Autodesk Inventor part; units mm, degrees
ref_plane "YZ Plane" through (0, 0, 0) normal (1, 0, 0) x (0, 1, 0)
ref_plane "XZ Plane" through (0, 0, 0) normal (0, 1, 0) x (-1, 0, 0)
ref_plane "XY Plane" through (0, 0, 0) normal (0, 0, 1) x (1, 0, 0)
sketch "草圖1" plane through (0, 0, 0) normal (0, 0, 1) x (1, 0, 0)
  line L0 (0, 0) -> (0, 7)
  line L1 (0, 7) -> (3.3317, 9.2136)
  line L2 (3.3317, 9.2136) -> (4.2133, 8)
  line L3 (4.2133, 8) -> (4.2133, 0)
  line L4 (4.2133, 0) -> (0, 0)
  dimension "d0" = 7
  dimension "d1" = 4
  dimension "d2" = 1.5
  dimension "d3" = 8
extrude "擠出1" add sketch "草圖1" along normal blind 5.3
sketch "草圖2" plane through (0, 0, 0) normal (-1, 0, 0) x (0, 0, 1)
  line L0 (1, 2.25) -> (4.3, 2.25)
  line L1 (4.4, 2.35) -> (4.4, 5.65)
  line L2 (4.3, 5.75) -> (1, 5.75)
  line L3 (0.9, 5.65) -> (0.9, 2.35)
  line L4 (0.9, 2.25) -> (4.4, 5.75) construction
  line L5 (4.4, 2.25) -> (0.9, 5.75) construction
  line L6 (1.2, 5.55) -> (2.2, 5.55)
  line L7 (2.3, 5.45) -> (2.3, 4.45)
  line L8 (2.2, 4.35) -> (1.2, 4.35)
  line L9 (1.1, 4.45) -> (1.1, 5.45)
  line L10 (1.1, 5.55) -> (2.3, 4.35) construction
  line L11 (2.3, 5.55) -> (1.1, 4.35) construction
  line L12 (3.1, 4.35) -> (4.1, 4.35)
  line L13 (4.2, 4.45) -> (4.2, 5.45)
  line L14 (4.1, 5.55) -> (3.1, 5.55)
  line L15 (3, 5.45) -> (3, 4.45)
  line L16 (3, 4.35) -> (4.2, 5.55) construction
  line L17 (4.2, 4.35) -> (3, 5.55) construction
  line L18 (3.1, 3.65) -> (4.1, 3.65)
  line L19 (4.2, 3.55) -> (4.2, 2.55)
  line L20 (4.1, 2.45) -> (3.1, 2.45)
  line L21 (3, 2.55) -> (3, 3.55)
  line L22 (3, 3.65) -> (4.2, 2.45) construction
  line L23 (4.2, 3.65) -> (3, 2.45) construction
  line L24 (1.2, 2.45) -> (2.2, 2.45)
  line L25 (2.3, 2.55) -> (2.3, 3.55)
  line L26 (2.2, 3.65) -> (1.2, 3.65)
  line L27 (1.1, 3.55) -> (1.1, 2.55)
  line L28 (1.1, 2.45) -> (2.3, 3.65) construction
  line L29 (2.3, 2.45) -> (1.1, 3.65) construction
  arc A0 (1, 5.75) -> (0.9, 5.65) centre (1, 5.65) ccw
  arc A1 (0.9, 2.35) -> (1, 2.25) centre (1, 2.35) ccw
  arc A2 (4.3, 2.25) -> (4.4, 2.35) centre (4.3, 2.35) ccw
  arc A3 (4.4, 5.65) -> (4.3, 5.75) centre (4.3, 5.65) ccw
  arc A4 (4.2, 5.45) -> (4.1, 5.55) centre (4.1, 5.45) ccw
  arc A5 (4.1, 4.35) -> (4.2, 4.45) centre (4.1, 4.45) ccw
  arc A6 (3, 4.45) -> (3.1, 4.35) centre (3.1, 4.45) ccw
  arc A7 (3.1, 5.55) -> (3, 5.45) centre (3.1, 5.45) ccw
  arc A8 (2.3, 5.45) -> (2.2, 5.55) centre (2.2, 5.45) ccw
  arc A9 (1.2, 5.55) -> (1.1, 5.45) centre (1.2, 5.45) ccw
  arc A10 (1.1, 4.45) -> (1.2, 4.35) centre (1.2, 4.45) ccw
  arc A11 (2.2, 4.35) -> (2.3, 4.45) centre (2.2, 4.45) ccw
  arc A12 (2.3, 3.55) -> (2.2, 3.65) centre (2.2, 3.55) ccw
  arc A13 (2.2, 2.45) -> (2.3, 2.55) centre (2.2, 2.55) ccw
  arc A14 (1.1, 2.55) -> (1.2, 2.45) centre (1.2, 2.55) ccw
  arc A15 (1.2, 3.65) -> (1.1, 3.55) centre (1.2, 3.55) ccw
  arc A16 (3.1, 3.65) -> (3, 3.55) centre (3.1, 3.55) ccw
  arc A17 (4.2, 3.55) -> (4.1, 3.65) centre (4.1, 3.55) ccw
  arc A18 (4.1, 2.45) -> (4.2, 2.55) centre (4.1, 2.55) ccw
  arc A19 (3, 2.55) -> (3.1, 2.45) centre (3.1, 2.55) ccw
  point P0 (2.65, 4)
  point P1 (1.7, 4.95)
  point P2 (3.6, 4.95)
  point P3 (3.6, 3.05)
  point P4 (1.7, 3.05)
  dimension "d7" = 3.5
  dimension "d8" = 3.5
  dimension "d9" = 1.2
  dimension "d10" = 1.2
  dimension "d11" = 0.2
  dimension "d12" = 0.1
  dimension "d13" = 0.1
extrude "擠出2" add sketch "草圖2" along normal blind 0.2
extrude "擠出3" cut sketch "草圖2" against normal blind 0.1 contours L6 A8 L7 A11 L8 A10 L9 A9 | A6 L15 A7 L14 A4 L13 A5 L12 | L18 A17 L19 A18 L20 A19 L21 A16 | A14 L27 A15 L26 A12 L25 A13 L24
sketch "草圖3" plane through (0, 0, 0) normal (0, -1, 0) x (1, 0, 0)
  line L0 (4.2133, 0) -> (4.2133, 5.3)
  line L1 (4.2133, 0.2) -> (0.2, 0.2)
  line L2 (0.2, 0.2) -> (0.2, 5.1)
  line L3 (0.2, 5.1) -> (4.2133, 5.1)
  line L4 (4.2133, 5.1) -> (4.2133, 0.2)
  line L5 (0, 0) -> (4.2133, 0)
  line L6 (0, 0) -> (0, 5.3)
  line L7 (0, 5.3) -> (4.2133, 5.3)
  dimension "d18" = 0.2
  dimension "d19" = 0.2
  dimension "d20" = 0.2
extrude "擠出4" add sketch "草圖3" along normal blind 3 contours L1 L2 L3 L0
sketch "草圖4" plane through (0.2, 0, 5.1) normal (0, 0, 1) x (1, 0, 0)
  line L0 (4.0133, 0) -> (0, 0)
  line L1 (0, 0) -> (4.0133, -3)
  line L2 (0, -3) -> (4.0133, -3)
  line L3 (4.0133, -3) -> (0, -3)
  line L4 (0, -3) -> (0, 0)
  point P0 (-0.2, 0)
extrude "擠出5" cut sketch "草圖4" against normal up to surface (4.9 mm away)
properties part number "頭 小小屋"
Design review of the part built by this model. Coordinates are the model's own, in mm. A direction names the side the tool comes from. Round coordinates to 2 decimals unless told otherwise and drop trailing zeros. Write each loop counter-clockwise with the first axis right and the second up, starting at its lowest first coordinate (ties: lowest second). Pieces come first, ordered by that corner, then holes. Notation, with made-up numbers: (17, -1.75) - (32, -1.75) arc R22 ccw to (32, 17.25) - close; hole circle Ø8 at (83, 8.5). An arc over 180 degrees is marked (long way). Use a Markdown table: item, result. Add a question column.
1. Wall thickness on probe 1 along Y at (x, z) = (0.05, 1.8); probe 2 along X at (y, z) = (5.25, 4.6); probe 3 along Z at (x, y) = (2.7, -0.25): over which ranges is each line inside the solid? List them lowest first.
2. We need section B-B (z = 3.8). State the section outline as (x, y) points, then the cut area to 3 significant figures.
3. For faces 4 (the face through (0.1, 3, 4)), 5 (the face through (3, -1, 0.2)), 6 (the face through (3, -1, 5.1)), list the 3-axis set-ups (+Z, -Z, +X, -X, +Y, -Y) from which the entire face can be reached by the end or side of a thin tool; tool diameter is ignored.
4. We need section A-A (y = 5.25). State the section outline as (x, z) points, then the cut area to 3 significant figures.
5. Clearance check with a flat-ended pin moving along its axis: pin 1 (2 mm diameter, centred on x = 1.5, z = 2.5, fed in from +Y). State where the tip first meets the part, or that it passes through.
6. Mouldability with a two-part tool opening along Y and no side actions: class faces 1 (the face through (-0.2, 4, 3)), 2 (the face through (1.64, 8.09, 2.61)), 3 (the face through (0.1, 5, 2)) as +Y half, -Y half, draft (parallel to the pull), parting line (faces both ways), or undercut.
7. We need section C-C (x = 0.85). State the section outline as (y, z) points.
8. We need section D-D (x = 2.4). State the section outline as (y, z) points.
Output:
| question | item | result |
|---|---|---|
| 1 | probe 1 | y = 0 to 2.45, 3.65 to 4.35, 5.55 to 7.03 |
| 1 | probe 2 | x = 0 to 4.21 |
| 1 | probe 3 | z = 0.2 to 5.1 |
| 2 | outline | (-0.2, 2.25) - (0, 2.25) - (0, 0) - (0.2, 0) - (4.21, -3) - (4.21, 8) - (3.33, 9.21) - (0, 7) - (0, 5.75) - (-0.2, 5.75) - (-0.2, 5.55) - (0.1, 5.55) - (0.1, 4.35) - (-0.2, 4.35) - (-0.2, 3.65) - (0.1, 3.65) - (0.1, 2.45) - (-0.2, 2.45) - close |
| 2 | area | 40.6 mm2 |
| 3 | face 4 | -X |
| 3 | face 5 | -Z, +X, -X, -Y |
| 3 | face 6 | +Z, +X, -X, -Y |
| 4 | outline | (-0.2, 0.9) - (0, 0.9) - (0, 0) - (4.21, 0) - (4.21, 5.3) - (0, 5.3) - (0, 4.4) - (-0.2, 4.4) - (-0.2, 4.2) - (0.1, 4.2) - (0.1, 3) - (-0.2, 3) - (-0.2, 2.3) - (0.1, 2.3) - (0.1, 1.1) - (-0.2, 1.1) - close |
| 4 | area | 22.3 mm2 |
| 5 | pin 1 | stops at y = 8.66 |
| 6 | face 1 | draft |
| 6 | face 2 | +Y half |
| 6 | face 3 | undercut |
| 7 | outline | (-0.49, 0.2) - (0, 0.2) - (0, 0) - (7.56, 0) - (7.56, 5.3) - (0, 5.3) - (0, 5.1) - (-0.49, 5.1) - close |
| 8 | outline | (-1.64, 0.2) - (0, 0.2) - (0, 0) - (8.59, 0) - (8.59, 5.3) - (0, 5.3) - (0, 5.1) - (-1.64, 5.1) - close |
